Work out the finished part from the listing and answer in its coordinate system (mm). A direction names the side the tool comes from. Coordinates: 2 decimals unless noted, no trailing zeros. Write each loop counter-clockwise with the first axis right and the second up, starting at its lowest first coordinate (ties: lowest second). Pieces come first, ordered by that corner, then holes. Notation, with made-up numbers: (-34.75, -28.75) - (2.25, -28.75) arc R15 ccw to (2.25, -13.75) - close; hole circle Ø8 at (87, 53.5). An arc over 180 degrees is marked (long way). Use one line per item in the form item = value. Start each with the question number.
Item 1: Given pin 1 (1 mm diameter, centred on x = 1.5, z = 19.5, fed in from -Y); pin 2 (3 mm diameter, centred on y = 0.5, z = 21, fed in from +X), each flat-ended and moving along its own axis, determine where each tip first touches the part or whether it passes through.
Item 2: A cutting plane is placed at C-C (y = -1.95). Write down the section's boundary in (x, z), then the cut area to 3 significant figures.
Item 3: For faces 5 (the flat face through (2.155, -1.267, 8.874)), 6 (the cylindrical face through (-1.5, 0.07, 21.94)), determine the directions among +Z, -Z, +X, -X, +Y, -Y from which every point of the face is accessible in a straight line to the end or side of a thin tool.
Item 4: A cutting plane is placed at A-A (z = 4). Write down the section's boundary in (x, y).
Item 5: A cutting plane is placed at B-B (z = 11.5). Write down the section's boundary in (x, y), then the cut area to 3 significant figures.
Item 6: A cutting plane is placed at D-D (x = 2.55). Write down the section's boundary in (y, z), then the cut area to 3 significant figures.
Item 7: Determine the mould class of faces 1 (the cylindrical face through (-0.27, -1.22, 4.06)), 2 (the flat face through (1.24, 1.15, 18)), 3 (the flat face through (-2.155, 1.267, 8.874)), 4 (the conical face through (0.05, -0.21, 8.62)) for opening direction X: released by +X, released by -X, zero draft, split by the parting line, or undercut.
Item 8: Consider probe 1 along Y at (x, z) = (0, 6); probe 2 along Z at (x, y) = (0.6, -1.75); probe 3 along Y at (x, z) = (-0.55, 5). Determine where each line is inside the solid, lowest interval first.
from build123d import *

# Parameters (mm, degrees)
BOSS_EXTRUDE1_DEPTH       = 18
SKETCH2_R                 = 1.5
BOSS_EXTRUDE2_DEPTH       = 8
M3X0_5_TAPPED_HOLE1_D     = 2.5
M3X0_5_TAPPED_HOLE1_DEPTH = 8
M3X0_5_TAPPED_HOLE1_TIP   = 0.751075774


with BuildPart() as part:
    # Sketch1 → Boss-Extrude1 (new body)
    with BuildSketch(Plane.XY):
        Polygon((-1.443375673, 2.5), (-2.886751346, 0), (-1.443375673, -2.5), (1.443375673, -2.5), (2.886751346, 0), (1.443375673, 2.5), align=None)
    extrude(amount=BOSS_EXTRUDE1_DEPTH)

    # Sketch2 → Boss-Extrude2 (add)
    with BuildSketch(Plane.XY.offset(18)):
        Circle(SKETCH2_R)
    extrude(amount=BOSS_EXTRUDE2_DEPTH)

    # M3x0.5 Tapped Hole1
    with Locations(Plane(origin=(0, 0, 0), x_dir=(-1, 0, 0), z_dir=(0, 0, -1))):
        with Locations((0, 0)):
            Hole(M3X0_5_TAPPED_HOLE1_D / 2, depth=M3X0_5_TAPPED_HOLE1_DEPTH)
            with Locations((0, 0, -(M3X0_5_TAPPED_HOLE1_DEPTH + M3X0_5_TAPPED_HOLE1_TIP / 2))):  # 118° drill point
                Cone(0, M3X0_5_TAPPED_HOLE1_D / 2, M3X0_5_TAPPED_HOLE1_TIP, mode=Mode.SUBTRACT)


solid = part.part
Answer:
q1.pin_1 = -1.12
q1.pin_2 = 1.5
q2.outline = (-1.76, 0) - (1.76, 0) - (1.76, 18) - (-1.76, 18) - close
q2.area = 63.4 mm²
q3.face_5 = +Z, -Z, +X, -Y
q3.face_6 = +Z
q4.outline = (-2.89, 0) - (-1.44, -2.5) - (1.44, -2.5) - (2.89, 0) - (1.44, 2.5) - (-1.44, 2.5) - close; hole circle Ø2.5 at (0, 0)
q5.outline = (-2.89, 0) - (-1.44, -2.5) - (1.44, -2.5) - (2.89, 0) - (1.44, 2.5) - (-1.44, 2.5) - close
q5.area = 21.7 mm²
q6.outline = (-0.58, 0) - (0.58, 0) - (0.58, 18) - (-0.58, 18) - close
q6.area = 21.0 mm²
q7.face_1 = undercut
q7.face_2 = zero draft
q7.face_3 = released by -X
q7.face_4 = undercut
q8.probe_1 = -2.5 to -1.25, 1.25 to 2.5
q8.probe_2 = 0 to 18
q8.probe_3 = -2.5 to -1.12, 1.12 to 2.5
